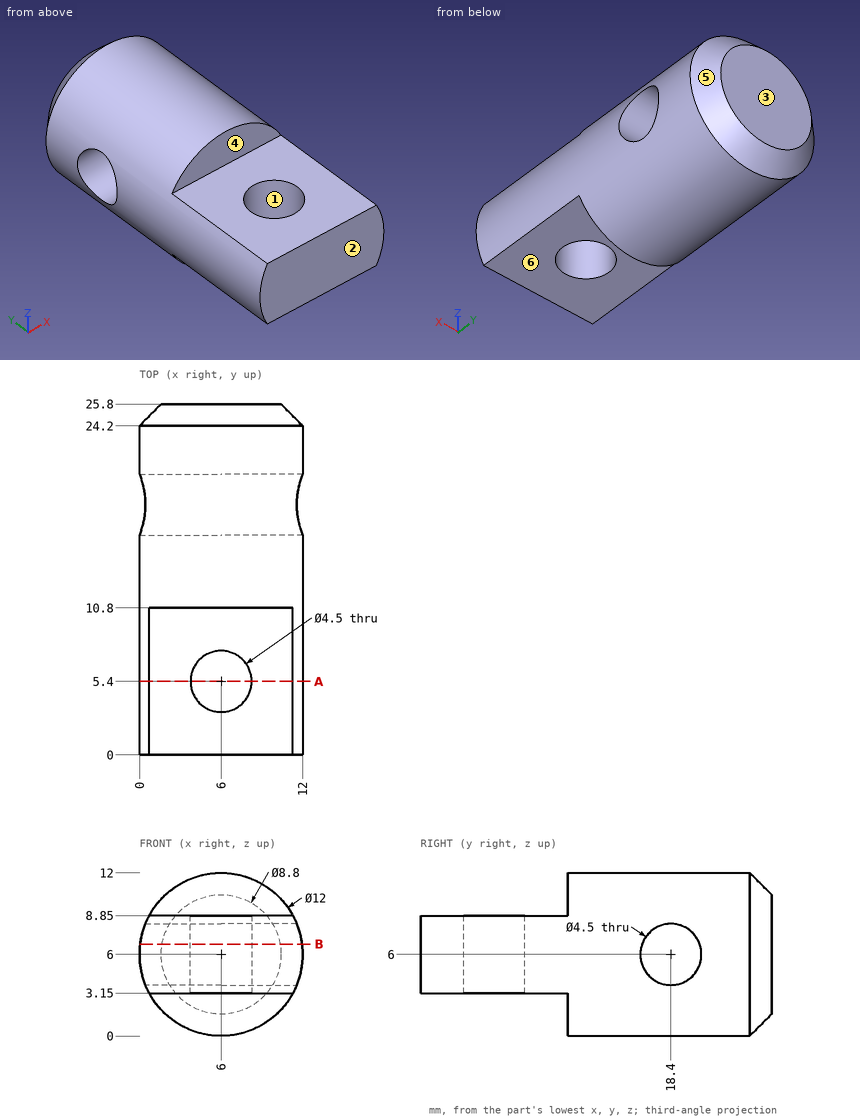
For this review, use the dimensioned drawing (mm, ordinates from the lowest corner) and the shaded views. A direction names the side the tool comes from. Coordinates: 2 decimals unless noted, no trailing zeros. Write each loop counter-clockwise with the first axis right and the second up, starting at its lowest first coordinate (ties: lowest second). Pieces come first, ordered by that corner, then holes. Notation, with made-up numbers: (-22, 75) - (-16, 75) arc R25 ccw to (-16, 106) - close; hole circle Ø6 at (10, -22.75). An arc over 180 degrees is marked (long way). One line per item, written item: value.
1) Add section B-B (z = 6.75). Give the number of separate pieces and of enclosed holes in the cut face, plus the area to 3 significant figures.
Answer sheet:
separate pieces: 2
enclosed holes: 1
area: 238 mm2
2) Add section A-A (y = 5.4). State the section outline as (x, z) points, plus the area to 3 significant figures.
Answer sheet:
outline: (0.72, 3.15) - (3.75, 3.15) - (3.75, 8.85) - (0.72, 8.85) arc R6 ccw to start; (8.25, 3.15) - (11.28, 3.15) arc R6 ccw to (11.28, 8.85) - (8.25, 8.85) - close
area: 40.1 mm2
3) To check wall thickness, follow probe 1 along Y at (x, z) = (3, 6); probe 2 along Y at (x, z) = (4, 6); probe 3 along Y at (x, z) = (3.75, 9.25). State the ranges of each line that lie inside material, in increasing order.
Answer sheet:
probe 1: y = 0 to 16.15, 20.65 to 25.8
probe 2: y = 0 to 4.37, 6.43 to 16.15, 20.65 to 25.8
probe 3: y = 10.8 to 25.8
4) For the marked faces 4, 5 and 6, list the 3-axis set-ups (+Z, -Z, +X, -X, +Y, -Y) from which the entire face can be reached by the end or side of a thin tool; tool diameter is ignored.
Answer sheet:
face 4: +Z, +X, -X, -Y
face 5: +Y
face 6: -Z, +X, -X, -Y
5) Mouldability with a two-part tool opening along Y and no side actions: class the marked faces 1, 2 and 3 as +Y half, -Y half, draft (parallel to the pull), parting line (faces both ways), or undercut.
Answer sheet:
face 1: undercut
face 2: -Y half
face 3: +Y half
6) Insertion check: pin 1 (6 mm diameter, centred on y = 4.5, z = 2, fed in from -X); pin 2 (4 mm diameter, centred on y = 18.4, z = 6, fed in from +X); pin 3 (5 mm diameter, centred on x = 6, y = 5.4, fed in from -Z); pin 4 (1.5 mm diameter, centred on y = 13, z = 2.5, fed in from -X). Each pin has a flat end and moves straight along its axis. Give the tip position at first contact, or say it passes through.
Answer sheet:
pin 1: stops at x = 0.08
pin 2: passes through
pin 3: stops at z = 3.15
pin 4: stops at x = 0.67
